Geometry check sheet. Reference: the model listing, model coordinates, mm. Face numbers are marked on the shaded views. A direction names the side the tool comes from. Round coordinates to 2 decimals unless told otherwise and drop trailing zeros. Order: outer loops, then holes, each group sorted by start corner. A loop starts at its lowest first (then second) coordinate and runs counter-clockwise, first axis right, second up.
```python
from build123d import *

# Parameters (mm, degrees)
SKETCH_1_W          = 28
SKETCH_1_H          = 35
EXTRUDE_1_DEPTH     = 4.5
SKETCH_2_W          = 28
SKETCH_2_H          = 35
EXTRUDE_2_DEPTH     = 4.5
EXTRUDE_3_DEPTH     = 2.6
CUT_EXTRUDE_1_DEPTH = 38.848381736
CUT_EXTRUDE_2_DEPTH = 49.489689626
FILLET_1_R          = 1


with BuildPart() as part:
    # 草图1 → 凸台-拉伸1 (new body)
    with BuildSketch(Plane.XY):
        Rectangle(SKETCH_1_W, SKETCH_1_H)
    extrude(amount=EXTRUDE_1_DEPTH)

    # 草图2 → 凸台-拉伸2 (add)
    with BuildSketch(Plane.XZ.offset(17.5)):
        with Locations((0, 17.5)):
            Rectangle(SKETCH_2_W, SKETCH_2_H)
    extrude(amount=-EXTRUDE_2_DEPTH)

    # 草图3 → 凸台-拉伸3 (add)
    with BuildSketch(Plane.ZY.offset(14)):
        Polygon((4.5, 17.5), (6.5, 17.5), (6.5, 12.5), (30, -11), (35, -11), (35, -13), (4.5, -13), align=None)
    extrude_3 = extrude(amount=-EXTRUDE_3_DEPTH)

    # 镜向1: 凸台-拉伸3 across plane
    add(extrude_3.mirror(Plane(origin=(0, 0, 0), x_dir=(0, 0, 1), z_dir=(1, 0, 0))))

    # 草图5 → 切除-拉伸1 (cut, through all)
    with BuildSketch(Plane.XY.offset(4.5)):
        with BuildLine():
            Line((-3.4, -5), (-3.4, 4))
            ThreePointArc((-3.4, 4), (0, 7.4), (3.4, 4))
            Line((3.4, 4), (3.4, -5))
            ThreePointArc((3.4, -5), (0, -8.4), (-3.4, -5))
        make_face()
    extrude(amount=-CUT_EXTRUDE_1_DEPTH, mode=Mode.SUBTRACT)

    # 草图6 → 切除-拉伸2 (cut, through all)
    with BuildSketch(Plane(origin=(0, -13, 0), x_dir=(1, 0, 0), z_dir=(0, 1, 0))):
        with BuildLine():
            Line((3.4, -12.5), (3.4, -21.5))
            ThreePointArc((3.4, -21.5), (0, -24.9), (-3.4, -21.5))
            Line((-3.4, -21.5), (-3.4, -12.5))
            ThreePointArc((-3.4, -12.5), (0, -9.1), (3.4, -12.5))
        make_face()
    extrude(amount=-CUT_EXTRUDE_2_DEPTH, mode=Mode.SUBTRACT)

    # 圆角1
    fillet_1_edges = [part.edges().sort_by_distance(p)[0] for p in [
        (-12.7, 17.5, 6.5),
        (-12.7, -11, 35),
        (12.7, -11, 35),
        (12.7, 17.5, 6.5),
    ]]
    fillet(fillet_1_edges, radius=FILLET_1_R)


solid = part.part
```
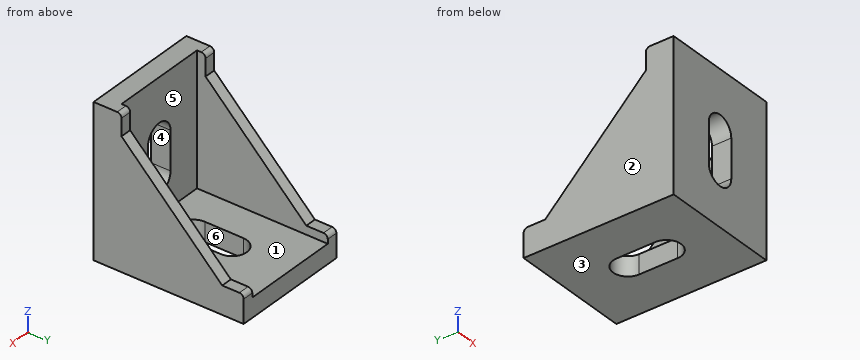
(1) Sectioned sample at A-A, the plane y = 2. Record the cut outline in (x, z), and give its area (3 significant figures).
Returned:
outline: (-14, 0) - (-3.4, 0) - (-3.4, 4.5) - (-11.4, 4.5) - (-11.4, 17) - (-14, 17) - close; (3.4, 0) - (14, 0) - (14, 17) - (11.4, 17) - (11.4, 4.5) - (3.4, 4.5) - close
area: 160 mm2
(2) Set-up check for the marked faces 4, 5 and 6: record each of +Z, -Z, +X, -X, +Y, -Y from which the full face is reachable in a straight line by a thin tool's end or side.
Returned:
face 4: +Y, -Y
face 5: +Z, +Y
face 6: +Z, -Z
(3) Draft check along X on the marked faces 1, 2 and 3. Enter one of: released by +X, released by -X, zero draft, split by the parting line, or undercut.
Returned:
face 1: undercut
face 2: released by -X
face 3: zero draft
(4) Sectioned sample at B-B, the plane z = 19.5. Record the cut outline in (x, y), and give its area (3 significant figures).
Returned:
outline: (-14, -17.5) - (-3.4, -17.5) - (-3.4, -13) - (-11.4, -13) - (-11.4, -0.5) - (-14, -0.5) - close; (3.4, -17.5) - (14, -17.5) - (14, -0.5) - (11.4, -0.5) - (11.4, -13) - (3.4, -13) - close
area: 160 mm2
(5) Depth check by flat-ended pin: P1, Ø3, axis at x = 13, z = 32.5, coming from the +Y side; P2, Ø2, axis at x = 0.5, z = 19, coming from the -Y side; P3, Ø2, axis at x = 12, y = 14.5, coming from the +Z side; P4, Ø10, axis at x = 6, z = 18, coming from the +Y side. Enter the tip coordinate at first touch or a pass-through.
Returned:
P1: stops at y = -11
P2: passes through
P3: stops at z = 6.5
P4: stops at y = -13
(6) Sectioned sample at D-D, the plane y = -14.5. Record the cut outline in (x, z), and give its area (3 significant figures).
Returned:
outline: (-14, 0) - (14, 0) - (14, 35) - (-14, 35) - close; hole (-3.4, 12.5) arc R3.4 ccw to (3.4, 12.5) - (3.4, 21.5) arc R3.4 ccw to (-3.4, 21.5) - close
area: 882 mm2
(7) Material ranges on line 1 (X direction, y = -9, z = 24); line 2 (Y direction, x = 5.25, z = 17); line 3 (Z direction, x = 8.5, y = 13), recorded low to high.
Returned:
line 1: x = -14 to -11.4, 11.4 to 14
line 2: y = -17.5 to -13
line 3: z = 0 to 4.5
(8) Sectioned sample at C-C, the plane x = 0. Record the cut outline in (y, z), and give its area (3 significant figures).
Returned:
outline: (-17.5, 0) - (-8.4, 0) - (-8.4, 4.5) - (-13, 4.5) - (-13, 9.1) - (-17.5, 9.1) - close; (-17.5, 24.9) - (-13, 24.9) - (-13, 35) - (-17.5, 35) - close; (7.4, 0) - (17.5, 0) - (17.5, 4.5) - (7.4, 4.5) - close
area: 153 mm2
